Autodesk Inventor part; units mm, degrees
ref_plane "YZ Plane" through (0, 0, 0) normal (1, 0, 0) x (0, 1, 0)
ref_plane "XZ Plane" through (0, 0, 0) normal (0, 1, 0) x (-1, 0, 0)
ref_plane "XY Plane" through (0, 0, 0) normal (0, 0, 1) x (1, 0, 0)
sketch "スケッチ1" plane through (0, 0, 0) normal (1, 0, 0) x (0, 1, 0)
  line L0 (0, 0) -> (0, 125) construction
  arc A0 (10.4476, 126.4665) -> (-10.542, 124.5901) centre (0, 125) ccw
  arc A1 (9.5221, 125.7296) -> (-7.8176, 119.5148) centre (0, 125) ccw construction
  line L1 (9.5221, 125.7296) -> (19.0442, 1.4592) construction
  line L2 (-7.8176, 119.5148) -> (-1.1797, 110.0544) construction
  arc A2 (-0.7923, 105.8489) -> (-1.1797, 110.0544) centre (-4.6587, 107.6133) ccw construction
  circle A3 centre (-4.6587, 107.6133) radius 4
  arc A4 (-4.5464, 108.0035) -> (-4.7566, 107.2192) centre (5.9664, 104.7663) ccw construction
  circle A5 centre (5.9664, 104.7663) radius 1.6 construction
  arc A6 (17.3156, 27.8342) -> (10.9958, -0.3023) centre (85.9675, -2.3638) ccw
  arc A7 (-10.9929, -0.3964) -> (10.9958, -0.3023) centre (0, 0) ccw
  arc A8 (-10.9929, -0.3964) -> (-17.5957, 27.7797) centre (-85.9441, -3.099) ccw
  line L3 (-15.1422, 75.5391) -> (-18.1148, 30.6464)
  line L4 (5.9664, 104.7663) -> (-4.6587, 107.6133) construction
  arc A9 (-18.742, 3.6807) -> (19.0442, 1.4592) centre (0, 0) ccw construction
  arc A10 (17.3156, 27.8342) -> (17.8229, 30.3321) centre (11.8235, 30.25) ccw
  arc A11 (-18.1148, 30.6464) -> (-17.5957, 27.7797) centre (-12.1279, 30.25) ccw
  line L5 (10.9958, -0.3023) -> (0, 0) construction
  line L6 (0, 0) -> (-10.9929, -0.3964) construction
  line L7 (9.4327, 35.2736) -> (6.8063, 69.5498)
  line L8 (-7.9258, 63.4396) -> (-9.7871, 35.3299)
  arc A12 (-6.8998, 31.221) -> (6.4814, 31.1048) centre (0, 55.25) ccw
  arc A13 (6.4814, 31.1048) -> (9.4327, 35.2736) centre (5.4444, 34.968) ccw
  arc A14 (-9.7871, 35.3299) -> (-6.8998, 31.221) centre (-5.7959, 35.0656) ccw
  arc A15 (-5.4818, 66.8639) -> (-7.9258, 63.4396) centre (-3.9346, 63.1753) ccw
  line L9 (-0.7923, 105.8489) -> (-13.5138, 77.9726) construction
  line L10 (-14.1444, 75.4731) -> (-19.3486, -3.1223) construction
  arc A16 (-13.5138, 77.9726) -> (-14.1444, 75.4731) centre (-7, 75) ccw construction
  arc A17 (-14.9577, 76.8059) -> (-15.1422, 75.5391) centre (-7, 75) ccw
  circle A18 centre (-4.6587, 107.6133) radius 6 construction
  arc A19 (6.9396, 102.6901) -> (7.8473, 106.0778) centre (-4.6587, 107.6133) ccw
  arc A20 (3.994, 103.9405) -> (4.6712, 106.4678) centre (-4.6587, 107.6133) ccw
  arc A21 (7.8473, 106.0778) -> (4.6712, 106.4678) centre (6.2593, 106.2728) ccw
  arc A22 (3.994, 103.9405) -> (6.9396, 102.6901) centre (5.4668, 103.3153) ccw
  line L11 (6.2593, 106.2728) -> (-4.6587, 107.6133) construction
  line L12 (-4.6587, 107.6133) -> (5.4668, 103.3153) construction
  line L13 (11.8235, 30.25) -> (-12.1279, 30.25) construction
  arc A23 (6.8063, 69.5498) -> (1.7829, 71.5275) centre (3.8151, 69.3206) ccw
  arc A24 (-5.4818, 66.8639) -> (1.7829, 71.5275) centre (-15.1521, 89.9179) ccw
  arc A25 (17.8229, 30.3321) -> (10.4476, 126.4665) centre (-749.1865, 19.8382) ccw
  line L14 (12.0148, 125.9206) -> (21.5369, 1.6502) construction
  line L15 (11.4747, 113.335) -> (17.1037, 39.8734) construction
  arc A26 (-14.9577, 76.8059) -> (-10.542, 124.5901) centre (-194.0689, 117.4533) ccw
  line L16 (0, 125) -> (-4.6587, 107.6133) construction
  circle A27 centre (-7, 75) radius 8 construction
  line L17 (3.8151, 69.3206) -> (-3.9346, 63.1753) construction
  line L18 (-7, 75) -> (-0.0598, 66.2479) construction
  point P0 (-14.406, 86.6566)
  point P1 (17.9231, 29.1792)
  point P2 (-14.4228, 86.4034)
  point P3 (-9.9857, 32.3309)
  point P4 (9.6685, 32.1953)
  point P5 (7.074, 66.0557)
  dimension "d2" = 125
  dimension "d10" = 19.1
  dimension "d13" = 8
  dimension "d14" = 0.25
  dimension "d20" = 3.2
  dimension "d25" = 11
  dimension "d75" = 19.1
  dimension "d79" = 1
  dimension "d86" = 6
  dimension "d87" = 75
  dimension "d95" = 8
  dimension "d96" = 4
  dimension "d109" = 1
  dimension "d111" = 75
  dimension "d116" = 12
  dimension "d117" = 11
  dimension "d118" = 16
  dimension "d119" = 30.25
  dimension "d120" = 25
  dimension "d124" = 3
  dimension "d128" = 25
  dimension "d130" = 2.5
  dimension "d131" = 8
  dimension "d132" = 18
  dimension "d133" = 15
  dimension "d134" = 7
  dimension "d135" = 16
  dimension "d136" = 7.16
extrude "押し出し1" add sketch "スケッチ1" along normal blind 2
hole "穴1" at (0, 0, 0) direction (1, 0, 0) diameter 8 end through all counterbore diameter 9.3 counterbore depth 0.65
hole "穴2" at (0, -7, 75) direction (1, 0, 0) diameter 6 end through all counterbore diameter 7.3 counterbore depth 0.65
hole "穴3" at (0, 0, 125) direction (1, 0, 0) diameter 10 end through all counterbore diameter 11.3 counterbore depth 0.65
properties part number "UPPER_LEG_OUTER_FRAME"
Geometry: final body of the model. Coordinates: model frame, mm. A direction names the side the tool comes from. Coordinates: 2 decimals unless noted, no trailing zeros. Order: outer loops, then holes, each group sorted by start corner. A loop starts at its lowest first (then second) coordinate and runs counter-clockwise, first axis right, second up. Notation, with made-up numbers: (26.5, 37.25) - (78.5, 37.25) arc R27 cw to (78.5, 54.25) - close; hole circle Ø5 at (11.5, 83.5). An arc over 180 degrees is marked (long way). Return JSON: item names as keys, results as strings. Group by question number.
1. Cut plane B-B (z = 74). Output: boundary loops of the cut face in (x, y), plus the area to 3 significant figures.
2. Material intervals for line 1 along Z through (x, y) = (0.95, 1); line 2 along Y through (x, z) = (0.8, 104); line 3 along Z through (x, y) = (0.15, -3), sorted ascending. Write a range as [from, to].
3. Pin query (flat end, axial travel): pin 1 (3.5 mm diameter, centred on y = -8.5, z = 74.5, fed in from -X); pin 2 (6 mm diameter, centred on y = 0, z = 125, fed in from +X). Return the tip coordinate at first contact, or that it passes through.
4. Set-up query: faces 1 (the face through (0.65, 5, 127)), 2 (the face through (0.99, -11.15, 100.89)), 3 (the face through (0.99, 4.87, 72.13)), 4 (the face through (2, 8, 63)), 5 (the face through (0.986, 15.595, 79.189)). Return all of +Z, -Z, +X, -X, +Y, -Y with unobstructed straight access to the full face (end or side cutting, diameter ignored); none if empty.
5. Cut plane D-D (y = -13). Output: boundary loops of the cut face in (x, z), plus the area to 3 significant figures.
6. Cut plane C-C (z = 16). Output: boundary loops of the cut face in (x, y).
7. Cut plane A-A (x = 1.4). Output: boundary loops of the cut face in (y, z).
8. Pull-direction query (Z, two-part tool) for faces 6 (the face through (0.99, 8.73, 32.69)), 7 (the face through (1, 0, -11)), 8 (the face through (0, 8, 63)), 9 (the face through (0.65, -4, 74)); classes: pulls with the +Z half, pulls with the -Z half, needs draft (parallel to the pull), parting line crosses it, or undercut.
Resolved:
{
 "1": {"outline": "(0, -15.24) - (2, -15.24) - (2, -9.83) - (0.65, -9.83) - (0.65, -10.51) - (0, -10.51) - close; (0, -3.49) - (0.65, -3.49) - (0.65, -4.17) - (2, -4.17) - (2, 15.98) - (0, 15.98) - close", "area": "50.2 mm²"},
 "2": {"line 1": "z = [-10.95, -3.87], [3.87, 30.27], [70.84, 120.1], [129.9, 135.5]", "line 2": "y = [-10.9, -6.37], [-2.94, 4.02], [7.41, 13.26]", "line 3": "z = [-10.58, -3.55], [3.55, 30.43], [68.07, 103.97], [111.25, 120.21], [129.79, 135.11]"},
 "3": {"pin 1": "stops at x = 0.65", "pin 2": "passes through"},
 "4": {"face 1": "-X", "face 2": "+X, -X, -Y", "face 3": "+X, -X", "face 4": "+Z, -Z, +X, +Y, -Y", "face 5": "+Z, +X, -X, +Y"},
 "5": {"outline": "(0, 14.34) - (2, 14.34) - (2, 86.68) - (0, 86.68) - close", "area": "145 mm²"},
 "6": {"outline": "(0, -13.42) - (2, -13.42) - (2, 13.25) - (0, 13.25) - close"},
 "7": {"outline": "(-18.11, 30.65) arc R6 ccw to (-17.6, 27.78) arc R75 cw to (-10.99, -0.4) arc R11 ccw to (11, -0.3) arc R75 cw to (17.32, 27.83) arc R6 ccw to (17.82, 30.33) arc R767.08 ccw to (10.45, 126.47) arc R10.55 ccw to (-10.54, 124.59) arc R183.67 cw to (-14.96, 76.81) arc R8.16 ccw to (-15.14, 75.54) - close; hole circle Ø6 at (-7, 75); hole (-9.79, 35.33) arc R4 ccw to (-6.9, 31.22) arc R25 ccw to (6.48, 31.1) arc R4 ccw to (9.43, 35.27) - (6.81, 69.55) arc R3 ccw to (1.78, 71.53) arc R25 cw to (-5.48, 66.86) arc R4 ccw to (-7.93, 63.44) - close; hole circle Ø8 at (-4.66, 107.61); hole circle Ø10 at (0, 125); hole circle Ø8 at (0, 0); hole (3.99, 103.94) arc R1.6 ccw to (6.94, 102.69) arc R12.6 ccw to (7.85, 106.08) arc R1.6 ccw to (4.67, 106.47) arc R9.4 cw to start"},
 "8": {"face 6": "undercut", "face 7": "pulls with the -Z half", "face 8": "needs draft", "face 9": "undercut"}
}
